Design review of the part built by this model. Coordinates are the model's own, in mm. A direction names the side the tool comes from. Coordinates: 2 decimals unless noted, no trailing zeros. Loops run counter-clockwise (first coordinate to the right, second up) from the corner with the lowest first, then second, coordinate; pieces in that order, holes last. Notation, with made-up numbers: M 31,84 L 57,84 A21 cw 57,105 Z; hole C 81.5,71 d3. An arc over 180 degrees is marked long. Answer as a JSON object with one key per item and string values. Group by question number.
1. Consider section C-C (x = -4.5). State the section outline as (y, z) points.
2. Insertion check: pin 1 (1.5 mm diameter, centred on y = -28.5, z = 3, fed in from -X); pin 2 (2 mm diameter, centred on x = -14, y = -20.5, fed in from +Z); pin 3 (2.5 mm diameter, centred on x = -12, z = 3.5, fed in from +Y). Each pin has a flat end and moves straight along its axis. Give the tip position at first contact, or say it passes through.
3. Consider section A-A (z = 3.9). State the section outline as (x, y) points.
4. Consider section D-D (x = 15). Count the separate pieces of the cut face and the enclosed holes in it, then the cut area to 3 significant figures.
5. Machinability: for faces 4 (the flat face through (-25, -42.468, 1)), 5 (the flat face through (32.74, -21, 1)), 6 (the flat face through (-38.76, -21, 3)), 7 (the flat face through (-41.26, -21, 1)), 8 (the flat face through (-5, 15.85, 3)), which of the approach directions +Z, -Z, +X, -X, +Y, -Y give a long, thin tool a straight path to every point of the face, cutting with its end or side? Answer none if there is none.
6. Consider section B-B (y = -20.15). State the section outline as (x, z) points.
7. To check wall thickness, follow probe 1 along Y at (x, z) = (18.5, 0.95); probe 2 along Y at (x, z) = (-2, 3.85); probe 3 along X at (y, z) = (-30, 0.75). State the ranges of each line that lie inside material, in increasing order.
8. Draft analysis for pull direction Y (two halves, no side actions). For faces 1 (the flat face through (-26, -12, 2)), 2 (the flat face through (30.24, -21, 3)), 3 (the flat face through (16, -44.468, 1)), state which applies: +Y half, -Y half, draft (parallel to the pull), parting line (faces both ways), or undercut.
from build123d import *

# Parameters (mm, degrees)
SKIZZE1_W                       = 74
SKIZZE1_H                       = 81
AUFSATZ_LINEAR_AUSTRAGEN1_DEPTH = 2
SKIZZE2_W                       = 69
SKIZZE2_H                       = 76
SKIZZE2_W_2                     = 65
SKIZZE2_H_2                     = 72
AUFSATZ_LINEAR_AUSTRAGEN2_DEPTH = 3
SKIZZE3_R                       = 22.5
SKIZZE3_R_2                     = 15.5
SCHNITT_LINEAR_AUSTRAGEN3_DEPTH = 1.5
SKIZZE4_W                       = 10
SKIZZE4_H                       = 1
SCHNITT_LINEAR_AUSTRAGEN4_DEPTH = 3
SKIZZE5_W                       = 10
SKIZZE5_H                       = 1
SCHNITT_LINEAR_AUSTRAGEN5_DEPTH = 3


with BuildPart() as part:
    # Skizze1 → Aufsatz-Linear austragen1 (new body)
    with BuildSketch(Plane.XY):
        with Locations((-4.260212221, -20.15)):
            Rectangle(SKIZZE1_W, SKIZZE1_H)
    extrude(amount=AUFSATZ_LINEAR_AUSTRAGEN1_DEPTH)

    # Skizze2 → Aufsatz-Linear austragen2 (add)
    with BuildSketch(Plane.XY.offset(2)):
        with Locations((-4.260212221, -20.15)):
            Rectangle(SKIZZE2_W, SKIZZE2_H)
        with Locations((-4.260212221, -20.15)):
            Rectangle(SKIZZE2_W_2, SKIZZE2_H_2, mode=Mode.SUBTRACT)
    extrude(amount=AUFSATZ_LINEAR_AUSTRAGEN2_DEPTH)

    # Skizze3 → Schnitt-Linear austragen3 (cut)
    with BuildSketch(Plane.XY.offset(2)):
        with Locations((-4.260212221, -20.15)):
            Circle(SKIZZE3_R)
        with Locations((-4.260212221, -20.15)):
            Circle(SKIZZE3_R_2, mode=Mode.SUBTRACT)
    extrude(amount=-SCHNITT_LINEAR_AUSTRAGEN3_DEPTH, mode=Mode.SUBTRACT)

    # Skizze4 → Schnitt-Linear austragen4 (cut, through all)
    with BuildSketch(Plane.XY.offset(2)):
        with Locations((-24.731661751, -48.968325553)):
            Rectangle(SKIZZE4_W, SKIZZE4_H)
        with Locations((-24.731661751, -50.968325553)):
            Rectangle(SKIZZE4_W, SKIZZE4_H)
        with Locations((-24.731661751, -46.968325553)):
            Rectangle(SKIZZE4_W, SKIZZE4_H)
        with Locations((-24.731661751, -44.968325553)):
            Rectangle(SKIZZE4_W, SKIZZE4_H)
        with Locations((-24.731661751, -42.968325553)):
            Rectangle(SKIZZE4_W, SKIZZE4_H)
    extrude(amount=-SCHNITT_LINEAR_AUSTRAGEN4_DEPTH, mode=Mode.SUBTRACT)

    # Skizze5 → Schnitt-Linear austragen5 (cut, through all)
    with BuildSketch(Plane.XY.offset(2)):
        with Locations((16.209787779, -50.968325553)):
            Rectangle(SKIZZE5_W, SKIZZE5_H)
        with Locations((16.209787779, -48.968325553)):
            Rectangle(SKIZZE5_W, SKIZZE5_H)
        with Locations((16.209787779, -46.968325553)):
            Rectangle(SKIZZE5_W, SKIZZE5_H)
        with Locations((16.209787779, -44.968325553)):
            Rectangle(SKIZZE5_W, SKIZZE5_H)
        with Locations((16.209787779, -42.968325553)):
            Rectangle(SKIZZE5_W, SKIZZE5_H)
    extrude(amount=-SCHNITT_LINEAR_AUSTRAGEN5_DEPTH, mode=Mode.SUBTRACT)


solid = part.part
Findings below:
{
 "1": {"outline": "M -60.65,0 L 20.35,0 L 20.35,2 L 17.85,2 L 17.85,5 L 15.85,5 L 15.85,2 L 2.35,2 L 2.35,0.5 L -4.65,0.5 L -4.65,2 L -35.65,2 L -35.65,0.5 L -42.65,0.5 L -42.65,2 L -56.15,2 L -56.15,5 L -58.15,5 L -58.15,2 L -60.65,2 Z"},
 "2": {"pin 1": "stops at x = -38.76", "pin 2": "stops at z = 2", "pin 3": "stops at y = 17.85"},
 "3": {"outline": "M -38.76,-58.15 L 30.24,-58.15 L 30.24,17.85 L -38.76,17.85 Z; hole M -36.76,-56.15 L 28.24,-56.15 L 28.24,15.85 L -36.76,15.85 Z"},
 "4": {"separate pieces": "6", "enclosed holes": "0", "area": "129 mm^2"},
 "5": {"face 4": "+Z, -Z", "face 5": "+Z, -Z, +X, +Y, -Y", "face 6": "+Z, -X, +Y, -Y", "face 7": "+Z, -Z, -X, +Y, -Y", "face 8": "+Z"},
 "6": {"outline": "M -41.26,0 L 32.74,0 L 32.74,2 L 30.24,2 L 30.24,5 L 28.24,5 L 28.24,2 L 18.24,2 L 18.24,0.5 L 11.24,0.5 L 11.24,2 L -19.76,2 L -19.76,0.5 L -26.76,0.5 L -26.76,2 L -36.76,2 L -36.76,5 L -38.76,5 L -38.76,2 L -41.26,2 Z"},
 "7": {"probe 1": "y = -60.65 to -51.47, -50.47 to -49.47, -48.47 to -47.47, -46.47 to -45.47, -44.47 to -43.47, -42.47 to 20.35", "probe 2": "y = -58.15 to -56.15, 15.85 to 17.85", "probe 3": "x = -41.26 to -24.49, -16.23 to 7.71, 15.97 to 32.74"},
 "8": {"face 1": "undercut", "face 2": "draft", "face 3": "undercut"}
}
